Autodesk Fusion 360 part; units mm, degrees
sketch "Sketch1" plane through (0, 0, 0) normal (0, 1, 0) x (1, 0, 0)
  circle A0 centre (0, 0) radius 55 construction
  line L0 (48, 0) -> (48, 19.8823)
  line L1 (48, 19.8823) -> (19.8823, 48)
  line L2 (19.8823, 48) -> (-19.8823, 48)
  line L3 (-19.8823, 48) -> (-48, 19.8823)
  line L4 (-48, 19.8823) -> (-48, 0)
  line L5 (-48, 0) -> (48, 0) construction
  line L6 (0, -1.75) -> (0, -22.5) construction
  line L7 (50, 0) -> (50, 20.7107)
  line L8 (50, 20.7107) -> (20.7107, 50)
  line L9 (20.7107, 50) -> (-20.7107, 50)
  line L10 (-20.7107, 50) -> (-50, 20.7107)
  line L11 (-50, 20.7107) -> (-50, 0)
  line L12 (0, 0) -> (-54.6194, 22.6241) construction
  line L13 (60.5, 0) -> (60.5, 25.0599)
  line L14 (60.5, 25.0599) -> (25.0599, 60.5)
  line L15 (25.0599, 60.5) -> (-25.0599, 60.5)
  line L16 (-25.0599, 60.5) -> (-60.5, 25.0599)
  line L17 (-60.5, 25.0599) -> (-60.5, 0)
  line L18 (0, 60.5) -> (0, 50)
  line L19 (-50, 0) -> (-50, -5)
  line L20 (-50, -5) -> (-60.5, -5)
  line L21 (-60.5, -5) -> (-60.5, 0)
  line L22 (-6, 60.5) -> (-6, 50)
  point P0 (-55, 0)
  point P1 (-38.8909, -38.8909)
  point P2 (-54.6194, -22.6241)
  point P3 (0, -55)
  point P4 (-22.6241, -54.6194)
  point P5 (38.8909, -38.8909)
  point P6 (22.6241, -54.6194)
  point P7 (55, 0)
  point P8 (54.6194, -22.6241)
  point P9 (38.8909, 38.8909)
  point P10 (54.6194, 22.6241)
  point P11 (0, 55)
  point P12 (22.6241, 54.6194)
  point P13 (-38.8909, 38.8909)
  point P14 (-22.6241, 54.6194)
  dimension "d1" = 110
  dimension "d21" = 96
  dimension "d22" = 48
  dimension "d23" = 45
  dimension "d26" = 2
  dimension "d28" = 5
  dimension "d29" = 12.5
  dimension "d31" = 360
  dimension "d39" = 5
  dimension "d40" = 6
extrude "Extrude3" add sketch "Sketch1" along normal blind 3 contours L9 L10 L11 L15 L16 L17 L19 L20 L21 L22
hole "Hole2" at (-54.6194, 0, -22.6241) at (-38.8909, 0, -38.8909) at (-22.6241, 0, -54.6194) at (-55, 0, 0) direction (0, 1, 0) diameter 5.5 depth 5 tip angle 118
fillet "Fillet1" radius 10 2 edges at (-60.5, 1.5, -25.0599) (-25.0599, 1.5, -60.5)
fillet "Fillet2" radius 5 2 edges at (-50, 1.5, -20.7107) (-20.7107, 1.5, -50)
chamfer "Chamfer2" distance 1 angle 45 4 edges at (-50, 1.5, 5) (-60.5, 1.5, 5) (-6, 1.5, -50) (-6, 1.5, -60.5)
sketch "Sketch2" plane through (0, 3, 0) normal (0, 1, 0) x (-1, 0, 0)
  line L0 (6, -59.5) -> (7, -60.5)
  line L1 (7, -60.5) -> (20.9178, -60.5)
  arc A0 (20.9178, -60.5) -> (27.9889, -57.5711) centre (20.9178, -50.5) ccw
  line L2 (27.9889, -57.5711) -> (57.5711, -27.9889)
  arc A1 (57.5711, -27.9889) -> (60.5, -20.9178) centre (50.5, -20.9178) ccw
  line L3 (60.5, -20.9178) -> (60.5, 4)
  line L4 (60.5, 4) -> (59.5, 5)
  line L5 (59.5, 5) -> (51, 5)
  line L6 (51, 5) -> (50, 4)
  line L7 (50, 4) -> (50, -18.6396)
  arc A2 (48.5355, -22.1751) -> (50, -18.6396) centre (45, -18.6396) ccw
  line L8 (48.5355, -22.1751) -> (22.1751, -48.5355)
  arc A3 (18.6396, -50) -> (22.1751, -48.5355) centre (18.6396, -45) ccw
  line L9 (18.6396, -50) -> (7, -50)
  line L10 (7, -50) -> (6, -51)
  line L11 (6, -51) -> (6, -59.5)
  circle A4 centre (22.6241, -54.6194) radius 2.75
  circle A5 centre (54.6194, -22.6241) radius 2.75
  circle A6 centre (38.8909, -38.8909) radius 2.75
  circle A7 centre (55, 0) radius 2.75
Read the model definition and answer for the solid it produces. Units are mm, in the model's axes. A direction names the side the tool comes from. Round coordinates to 2 decimals unless told otherwise and drop trailing zeros. Write each loop counter-clockwise with the first axis right and the second up, starting at its lowest first coordinate (ties: lowest second). Pieces come first, ordered by that corner, then holes. Notation, with made-up numbers: (-16.75, 58) -> (21.25, 58) arc R36 ccw to (21.25, 92) -> close; hole circle Ø9 at (-1.5, -11.75). An arc over 180 degrees is marked (long way). Answer in a Markdown table with one row per item. Add a question column.
1) Which of the six approach directions +Z, -Z, +X, -X, +Y, -Y give full straight-line access (tool end or side, diameter ignored) to faces 5 (the face through (-13, 1, -50)), 6 (the face through (-24.69, 1.52, -59.76))?
2) Determine the mould class of faces 1 (the face through (-55, 1, 5)), 2 (the face through (-6, 1, -55)), 3 (the face through (-52.95, 1.52, -20.44)), 4 (the face through (-25.35, 1.52, -54.26)) for opening direction X: pulls with the +X half, pulls with the -X half, needs draft (parallel to the pull), parting line crosses it, or undercut.
3) Find section B-B, the plane y = 0.8. Determine the outline of the cut face in (x, z), and give its area (3 significant figures).
4) Find section A-A, the plane z = 0. Determine the outline of the cut face in (x, y), and give its area (3 significant figures).
5) Given P1, Ø1.5, axis at x = -13, y = 2, coming from the +Z side; P2, Ø1.5, axis at y = 2, z = -4.5, coming from the +X side, each flat-ended and moving along its own axis, determine where each tip first touches the part or whether it passes through.
6) Consider line 1 (Z direction, x = -55, y = 2.3); line 2 (Z direction, x = -54.5, y = 1); line 3 (X direction, y = 2.9, z = -6). Determine where each line is inside the solid, lowest interval first.
7) Find section C-C, the plane z = -53. Determine the outline of the cut face in (x, y), and give its area (3 significant figures).
8) Find section D-D, the plane z = -45. Determine the outline of the cut face in (x, y), and give its area (3 significant figures).
Findings below:
| question | item | result |
|---|---|---|
| 1 | face 5 | +Z, +X, +Y, -Y |
| 1 | face 6 | -Z, -X, +Y, -Y |
| 2 | face 1 | needs draft |
| 2 | face 2 | pulls with the +X half |
| 2 | face 3 | undercut |
| 2 | face 4 | undercut |
| 3 | outline | (-60.5, -20.92) arc R10 ccw to (-57.57, -27.99) -> (-27.99, -57.57) arc R10 ccw to (-20.92, -60.5) -> (-7, -60.5) -> (-6, -59.5) -> (-6, -51) -> (-7, -50) -> (-18.64, -50) arc R5 cw to (-22.18, -48.54) -> (-48.54, -22.18) arc R5 cw to (-50, -18.64) -> (-50, 4) -> (-51, 5) -> (-59.5, 5) -> (-60.5, 4) -> close; hole circle Ø5.5 at (-55, 0); hole circle Ø5.5 at (-54.62, -22.62); hole circle Ø5.5 at (-38.89, -38.89); hole circle Ø5.5 at (-22.62, -54.62) |
| 3 | area | 850 mm² |
| 4 | outline | (-60.5, 0) -> (-57.75, 0) -> (-57.75, 3) -> (-60.5, 3) -> close; (-52.25, 0) -> (-50, 0) -> (-50, 3) -> (-52.25, 3) -> close |
| 4 | area | 15.0 mm² |
| 5 | P1 | z = -50 |
| 5 | P2 | x = -50 |
| 6 | line 1 | -30.56 to -25.35, -19.9 to -2.75, 2.75 to 5 |
| 6 | line 2 | -31.06 to -25.37, -19.88 to -2.7, 2.7 to 5 |
| 6 | line 3 | -60.5 to -50 |
| 7 | outline | (-32.56, 0) -> (-24.85, 0) -> (-24.85, 3) -> (-32.56, 3) -> close; (-20.4, 0) -> (-6, 0) -> (-6, 3) -> (-20.4, 3) -> close |
| 7 | area | 66.3 mm² |
| 8 | outline | (-40.56, 0) -> (-25.71, 0) -> (-25.71, 3) -> (-40.56, 3) -> close |
| 8 | area | 44.5 mm² |
